```python
from build123d import *

# Parameters (mm, degrees)
SKETCH1_W            = 78
SKETCH1_H            = 21
BOSS_EXTRUDE1_DEPTH  = 7
CUT_EXTRUDE1_DEPTH   = 80.014239223
SKETCH3_W            = 70
SKETCH3_H            = 8
CUT_EXTRUDE2_DEPTH   = 6
CUT_EXTRUDE3_DEPTH   = 70
SKETCH5_W            = 68
SKETCH5_H            = 8
CUT_EXTRUDE4_DEPTH   = 41.831972766
BOSS_EXTRUDE2_DEPTH  = 12
MIRROR3_COPY_1_DEPTH = 12
BOSS_EXTRUDE3_DEPTH  = 4
SKETCH9_W            = 6.5
SKETCH9_H            = 3
CUT_EXTRUDE5_DEPTH   = 2
CUT_EXTRUDE6_DEPTH   = 2
SKETCH12_W           = 0.5
SKETCH12_H           = 6
CUT_EXTRUDE8_DEPTH   = 10.5
SKETCH13_W           = 4.001855858
SKETCH13_H           = 15
CUT_EXTRUDE9_DEPTH   = 2.3
SKETCH14_W           = 5
SKETCH14_H           = 1.5
CUT_EXTRUDE10_DEPTH  = 4


with BuildPart() as part:
    # Sketch1 → Boss-Extrude1 (new body)
    with BuildSketch(Plane(origin=(0, 0, 0), x_dir=(1, 0, 0), z_dir=(0, 1, 0))):
        Rectangle(SKETCH1_W, SKETCH1_H)
    extrude(amount=BOSS_EXTRUDE1_DEPTH)

    # Sketch2 → Cut-Extrude1 (cut, through all)
    with BuildSketch(Plane(origin=(39, 0, 0), x_dir=(0, 0, -1), z_dir=(1, 0, 0))):
        Polygon((10, 7), (10.5, 0), (10.5, 7), align=None)
        Polygon((-10, 7), (-10.5, 0), (-10.5, 7), align=None)
    extrude(amount=-CUT_EXTRUDE1_DEPTH, mode=Mode.SUBTRACT)

    # Sketch3 → Cut-Extrude2 (cut)
    with BuildSketch(Plane(origin=(0, 7, 0), x_dir=(1, 0, 0), z_dir=(0, 1, 0))):
        Rectangle(SKETCH3_W, SKETCH3_H)
    extrude(amount=-CUT_EXTRUDE2_DEPTH, mode=Mode.SUBTRACT)

    # Sketch4 → Cut-Extrude3 (cut)
    with BuildSketch(Plane(origin=(35, 0, 0), x_dir=(0, 0, -1), z_dir=(1, 0, 0))):
        with BuildLine():
            Line((4, 1), (4, 7))
            Line((4, 7), (8.5, 7))
            ThreePointArc((8.5, 7), (7.132310367, 3.338267225), (4, 1))
        make_face()
    cut_extrude3 = extrude(amount=-CUT_EXTRUDE3_DEPTH, mode=Mode.SUBTRACT)

    # Mirror1: Cut-Extrude3 across plane
    add(cut_extrude3.mirror(Plane.XY), mode=Mode.SUBTRACT)

    # Sketch5 → Cut-Extrude4 (cut, through all)
    with BuildSketch(Plane(origin=(0, 1, 0), x_dir=(1, 0, 0), z_dir=(0, 1, 0))):
        Rectangle(SKETCH5_W, SKETCH5_H)
    extrude(amount=-CUT_EXTRUDE4_DEPTH, mode=Mode.SUBTRACT)

    # Sketch6 → Boss-Extrude2 (add)
    with BuildSketch(Plane(origin=(26, 0, 0), x_dir=(0, 0, -1), z_dir=(1, 0, 0))):
        with BuildLine():
            Line((-10, 7), (-8.5, 7))
            ThreePointArc((-8.5, 7), (-8.740958247, 10.123493041), (-7.5, 13))
            ThreePointArc((-7.5, 13), (-9.343954985, 10.247481244), (-10, 7))
        make_face()
    boss_extrude2 = extrude(amount=-BOSS_EXTRUDE2_DEPTH)

    # Mirror2: Boss-Extrude2 across plane
    add(boss_extrude2.mirror(Plane(origin=(0, 0, 0), x_dir=(0, 0, 1), z_dir=(1, 0, 0))))

    # Mirror3: Boss-Extrude2 across plane
    add(boss_extrude2.mirror(Plane.XY))

    # Mirror3 copy 1 sketch → Mirror3 copy 1 (add)
    with BuildSketch(Plane.ZY.offset(26)):
        with BuildLine():
            Line((-10, 7), (-8.5, 7))
            ThreePointArc((-8.5, 7), (-8.740958247, 10.123493041), (-7.5, 13))
            ThreePointArc((-7.5, 13), (-9.343954985, 10.247481244), (-10, 7))
        make_face()
    extrude(amount=-MIRROR3_COPY_1_DEPTH)

    # Sketch8 → Boss-Extrude3 (add)
    with BuildSketch(Plane(origin=(39, 0, 0), x_dir=(0, 0, -1), z_dir=(1, 0, 0))):
        Polygon((-8, 15), (8, 15), (9.894572253, 8.304261216), (10, 7), (-10, 7), (-9.894572253, 8.304261216), align=None)
    boss_extrude3 = extrude(amount=-BOSS_EXTRUDE3_DEPTH)

    # Mirror4: Boss-Extrude3 across plane
    add(boss_extrude3.mirror(Plane(origin=(0, 0, 0), x_dir=(0, 0, 1), z_dir=(1, 0, 0))))

    # Sketch9 → Cut-Extrude5 (cut)
    with BuildSketch(Plane(origin=(39, 0, 0), x_dir=(0, 0, -1), z_dir=(1, 0, 0))):
        with Locations((0, 5.5)):
            Rectangle(SKETCH9_W, SKETCH9_H)
    cut_extrude5 = extrude(amount=-CUT_EXTRUDE5_DEPTH, mode=Mode.SUBTRACT)

    # Mirror5: Cut-Extrude5 across plane
    add(cut_extrude5.mirror(Plane(origin=(0, 0, 0), x_dir=(0, 0, 1), z_dir=(1, 0, 0))), mode=Mode.SUBTRACT)

    # Sketch11 → Cut-Extrude6 (cut)
    with BuildSketch(Plane.ZY.offset(-35)):
        Polygon((-2.5, 3.5), (2.5, 3.5), (2.5, 11.5), (3, 11.5), (3, 15), (-3, 15), (-3, 11.5), (-2.5, 11.5), align=None)
    cut_extrude6 = extrude(amount=-CUT_EXTRUDE6_DEPTH, mode=Mode.SUBTRACT)

    # Sketch12 → Cut-Extrude8 (cut)
    with BuildSketch(Plane(origin=(0, 11.5, 0), x_dir=(1, 0, 0), z_dir=(0, 1, 0))):
        with Locations((36.75, 0)):
            Rectangle(SKETCH12_W, SKETCH12_H)
    cut_extrude8 = extrude(amount=-CUT_EXTRUDE8_DEPTH, mode=Mode.SUBTRACT)

    # Sketch13 → Cut-Extrude9 (cut)
    with BuildSketch(Plane(origin=(39, 0, 0), x_dir=(0, 0, -1), z_dir=(1, 0, 0))):
        with Locations((0, 7.5)):
            Rectangle(SKETCH13_W, SKETCH13_H)
    cut_extrude9 = extrude(amount=-CUT_EXTRUDE9_DEPTH, mode=Mode.SUBTRACT)

    # Mirror6: Cut-Extrude6, Cut-Extrude8, Cut-Extrude9 across plane
    add(cut_extrude6.mirror(Plane(origin=(0, 0, 0), x_dir=(0, 0, 1), z_dir=(1, 0, 0))), mode=Mode.SUBTRACT)
    add(cut_extrude8.mirror(Plane(origin=(0, 0, 0), x_dir=(0, 0, 1), z_dir=(1, 0, 0))), mode=Mode.SUBTRACT)
    add(cut_extrude9.mirror(Plane(origin=(0, 0, 0), x_dir=(0, 0, 1), z_dir=(1, 0, 0))), mode=Mode.SUBTRACT)

    # Sketch14 → Cut-Extrude10 (cut)
    with BuildSketch(Plane.XZ):
        with Locations((0, 9.75)):
            Rectangle(SKETCH14_W, SKETCH14_H)
    cut_extrude10 = extrude(amount=-CUT_EXTRUDE10_DEPTH, mode=Mode.SUBTRACT)

    # Mirror7: Cut-Extrude10 across plane
    add(cut_extrude10.mirror(Plane.XY), mode=Mode.SUBTRACT)


solid = part.part
```
Read the model definition and answer for the solid it produces. Units are mm, in the model's axes. A direction names the side the tool comes from. Give positions to 0.01 mm unless a question says otherwise; leave off trailing zeros. Write each loop counter-clockwise with the first axis right and the second up, starting at its lowest first coordinate (ties: lowest second). Pieces come first, ordered by that corner, then holes. Notation, with made-up numbers: M 58,-22 L 77,-22 A25 ccw 77,8 Z; hole C -21,47.25 d9. An arc over 180 degrees is marked long. Put each result on its own line as item: value. Start each with the question number.
1. The part is cut by section A-A, the plane x = -32. Give the vertices of the cut face in (y, z).
2. Consider line 1 along X through (y, z) = (7.75, 8.75); line 2 along X through (y, z) = (12.5, 7); line 3 along X through (y, z) = (12.5, -2.25). Determine where each line is inside the solid, lowest interval first.
3. Which of the six approach directions +Z, -Z, +X, -X, +Y, -Y give full straight-line access (tool end or side, diameter ignored) to faces 5 (the flat face through (-38, 11, 2.001)), 6 (the flat face through (14, 9, 9)), 7 (the cylindrical face through (0.49, 3.383, 7.165))?
4. The part is cut by section B-B, the plane z = 0.5. Give the vertices of the cut face in (x, y), and give its area (3 significant figures).
5. The part is cut by section D-D, the plane x = 18. Give the vertices of the cut face in (y, z), and give its area (3 significant figures).
6. For a pull along Z with two mould halves and no side action, classify faces 1 (the flat face through (-39, 8, 6)), 2 (the flat face through (-38, 7, -3)), 3 (the flat face through (-37.03, 7.64, 9.95)), 4 (the flat face through (38, 2, 2.001)) as released by +Z, released by -Z, zero draft, split by the parting line, or undercut.
7. Each of these flat-tipped pins is pushed along its axis until it touches: pin 1 Ø0.6 at (x, z) = (36, -2.5) entering from +Y; pin 2 Ø0.6 at (x, y) = (-38.5, 10.5) entering from +Z; pin 3 Ø3 at (x, z) = (-6.5, -6) entering from +Y. Where does it stop, or does it pass through?
Final values:
1. outline: M 0,-10.5 L 7,-10 L 7,-8.5 A6.93 cw 1,-4 L 0,-4 Z; M 0,4 L 1,4 A6.93 cw 7,8.5 L 7,10 L 0,10.5 Z
2. line 1: x = -39 to -35, -26 to -14, 14 to 26, 35 to 39
2. line 2: x = -39 to -35, 35 to 39
2. line 3: x = -39 to -37, 37 to 39
3. face 5: +X, -X, +Y, -Y
3. face 6: +Z, -Z, +Y
3. face 7: none
4. outline: M -36.7,0 L -34,0 L -34,1 L -35,1 L -35,3.5 L -36.5,3.5 L -36.5,1 L -36.7,1 Z; M 34,0 L 36.7,0 L 36.7,1 L 36.5,1 L 36.5,3.5 L 35,3.5 L 35,1 L 34,1 Z
4. area: 12.9 mm²
5. outline: M 0,-10.5 L 7,-10 A8.53 ccw 13,-7.5 A6.53 cw 7,-8.5 A6.93 cw 1,-4 L 0,-4 Z; M 0,4 L 1,4 A6.93 cw 7,8.5 A6.53 cw 13,7.5 A8.53 ccw 7,10 L 0,10.5 Z
5. area: 57.7 mm²
6. face 1: zero draft
6. face 2: undercut
6. face 3: released by +Z
6. face 4: undercut
7. pin 1: stops at y = 11.5
7. pin 2: stops at z = 9.36
7. pin 3: stops at y = 3.88
